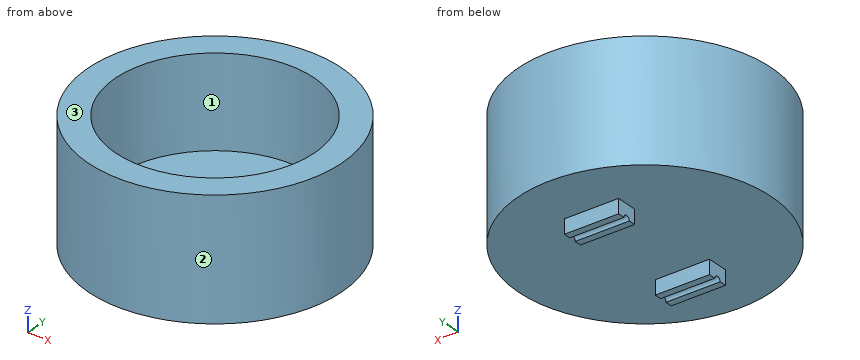
from build123d import *

# Parameters (mm, degrees)
SKETCH1_R           = 88.9
BOSS_EXTRUDE1_DEPTH = 83.8
SKETCH2_W           = 38.1
SKETCH2_H           = 15
BOSS_EXTRUDE2_DEPTH = 10
SKETCH4_R           = 2.5
CUT_EXTRUDE1_DEPTH  = 108.95
SKETCH5_R           = 2.5
CUT_EXTRUDE2_DEPTH  = 38.1
SKETCH6_R           = 69.85
CUT_EXTRUDE3_DEPTH  = 63.5


with BuildPart() as part:
    # Sketch1 → Boss-Extrude1 (new body)
    with BuildSketch(Plane.XY):
        Circle(SKETCH1_R)
    extrude(amount=BOSS_EXTRUDE1_DEPTH)

    # Sketch2 → Boss-Extrude2 (add)
    with BuildSketch(Plane(origin=(0, 0, 0), x_dir=(-1, 0, 0), z_dir=(0, 0, -1))):
        with Locations((0, 42.5)):
            Rectangle(SKETCH2_W, SKETCH2_H)
        with Locations((0, -42.5)):
            Rectangle(SKETCH2_W, SKETCH2_H)
    extrude(amount=BOSS_EXTRUDE2_DEPTH)

    # Sketch4 → Cut-Extrude1 (cut, through all)
    with BuildSketch(Plane(origin=(19.05, 0, 0), x_dir=(0, 0, -1), z_dir=(1, 0, 0))):
        with Locations((10, 42.5)):
            Circle(SKETCH4_R)
    extrude(amount=-CUT_EXTRUDE1_DEPTH, mode=Mode.SUBTRACT)

    # Sketch5 → Cut-Extrude2 (cut)
    with BuildSketch(Plane(origin=(19.05, 0, 0), x_dir=(0, 0, -1), z_dir=(1, 0, 0))):
        with Locations((10, -42.5)):
            Circle(SKETCH5_R)
    extrude(amount=-CUT_EXTRUDE2_DEPTH, mode=Mode.SUBTRACT)

    # Sketch6 → Cut-Extrude3 (cut)
    with BuildSketch(Plane.XY.offset(83.8)):
        Circle(SKETCH6_R)
    extrude(amount=-CUT_EXTRUDE3_DEPTH, mode=Mode.SUBTRACT)


solid = part.part
Can you work these out from the model? Positions are in its coordinate system, mm. Face numbers are marked on the shaded views. Give positions to 0.01 mm unless a question says otherwise; leave off trailing zeros. Loops run counter-clockwise (first coordinate to the right, second up) from the corner with the lowest first, then second, coordinate; pieces in that order, holes last. Notation, with made-up numbers: (17, -22) - (31, -22) arc R6 ccw to (31, -14) - close; hole circle Ø8 at (48.25, 63). An arc over 180 degrees is marked (long way). One line per item, written item: value.
(1) I'm going to push flat-ended pins straight in: pin 1 (11 mm diameter, centred on y = 46, z = -6, fed in from +X); pin 2 (8 mm diameter, centred on x = 4.5, z = -7.5, fed in from +Y); pin 3 (10 mm diameter, centred on x = 71, z = 33, fed in from +Y); pin 4 (12 mm diameter, centred on y = 3, z = 16, fed in from -X). Where does each tip first touch, or does it pass through?
Verdict:
pin 1: x = 19.05
pin 2: y = 50
pin 3: y = 59.56
pin 4: x = -88.9
(2) I need wall thicknesses on line 1 along Y through (x, z) = (0, 63.5); line 2 along Z through (x, y) = (-38, 70); line 3 along Z through (x, y) = (42, 28.5). Which ranges of each line are inside material? Lowest first, please.
Verdict:
line 1: -88.9 to -69.85, 69.85 to 88.9
line 2: 0 to 83.8
line 3: 0 to 20.3
(3) If we mould it in two halves opening along Y, with no side actions, what happens to the marked faces 1, 2 and 3? For each: released by +Y, released by -Y, zero draft, split by the parting line, or undercut.
Verdict:
face 1: undercut
face 2: split by the parting line
face 3: zero draft
(4) If we section it at A-A, the plane z = 62.5: List the corners of the cut face in (x, y) for me.
Verdict:
outline: circle Ø177.8 at (0, 0); hole circle Ø139.7 at (0, 0)
(5) If we section it at D-D, the plane z = 7: List the corners of the cut face in (x, y) for me.
Verdict:
outline: circle Ø177.8 at (0, 0)
(6) If we section it at C-C, the plane y = 0: List the corners of the cut face in (x, z) for me.
Verdict:
outline: (-88.9, 0) - (88.9, 0) - (88.9, 83.8) - (69.85, 83.8) - (69.85, 20.3) - (-69.85, 20.3) - (-69.85, 83.8) - (-88.9, 83.8) - close
(7) If we section it at B-B, the plane x = 0: List the corners of the cut face in (y, z) for me.
Verdict:
outline: (-88.9, 0) - (-50, 0) - (-50, -10) - (-45, -10) arc R2.5 cw to (-40, -10) - (-35, -10) - (-35, 0) - (35, 0) - (35, -10) - (40, -10) arc R2.5 cw to (45, -10) - (50, -10) - (50, 0) - (88.9, 0) - (88.9, 83.8) - (69.85, 83.8) - (69.85, 20.3) - (-69.85, 20.3) - (-69.85, 83.8) - (-88.9, 83.8) - close
